Source: CAD feature listing. Evaluate the final solid. Frame: model axes, mm. A direction names the side the tool comes from. Coordinates: 2 decimals unless noted, no trailing zeros. Order: outer loops, then holes, each group sorted by start corner. A loop starts at its lowest first (then second) coordinate and runs counter-clockwise, first axis right, second up.
Item 1: Contact query for flat-ended pins moving along their axis: P1, Ø1.5, axis at x = 4.5, z = -7, coming from the -Y side; P2, Ø2, axis at x = 8, z = -6.5, coming from the +Y side; P3, Ø10, axis at x = 4.5, z = -7, coming from the -Y side. Output: stop coordinate, or through.
Item 2: Section A-A on y = -29. Return the cut outline in (x, z), then the cut area to 3 significant figures.
Item 3: Ray query, line 1 (Z direction, x = -5.5, y = -33.5); line 2 (Y direction, x = 0.25, z = 6.75); line 3 (Z direction, x = -0.25, y = -3.5). Return the intervals inside material, ascending.
Item 4: Reachability of faces 1 (the flat face through (10, 0.381, -1)), 2 (the flat face through (-10, 0.381, -1)), 3 (the flat face through (6.2, 0, 2)) from +Z, -Z, +X, -X, +Y, -Y: full face, straight path, thin tool, end or side. Return the list, or none.
Autodesk Inventor part; units mm, degrees
ref_plane "YZ Plane" through (0, 0, 0) normal (1, 0, 0) x (0, 1, 0)
ref_plane "XZ Plane" through (0, 0, 0) normal (0, 1, 0) x (-1, 0, 0)
ref_plane "XY Plane" through (0, 0, 0) normal (0, 0, 1) x (1, 0, 0)
sketch "Sketch1" plane through (0, 0, 0) normal (0, 0, 1) x (1, 0, 0)
  line L0 (0, 0) -> (6.35, 0)
  line L1 (6.35, 0) -> (6.35, -44.45)
  line L2 (6.35, -44.45) -> (0, -44.45)
  line L3 (0, -44.45) -> (0, 0)
  dimension "d0" = 12.7
  dimension "d1" = 44.45
revolve "Revolution1" add sketch "Sketch1" angle 360 about axis through (0, -44.45, 0) along (0, 1, 0)
chamfer "Chamfer1" distance 3.175 angle 45 1 edges at (-6.35, -44.45, 0)
sketch "Sketch2" plane through (0, 0, 0) normal (0, 1, 0) x (1, 0, 0)
  circle A0 centre (0, 0) radius 9.525
  point P0 (0, 0)
  dimension "d6" = 19.05
extrude "Extrusion1" add sketch "Sketch2" along normal blind 6.35
sketch "Sketch3" plane through (0, 6.35, 0) normal (0, 1, 0) x (1, 0, 0)
  line L0 (10.9985, 0) -> (5.4993, -9.525)
  line L1 (5.4993, -9.525) -> (-5.4993, -9.525)
  line L2 (-5.4993, -9.525) -> (-10.9985, 0)
  line L3 (-10.9985, 0) -> (-5.4993, 9.525)
  line L4 (-5.4993, 9.525) -> (5.4993, 9.525)
  line L5 (5.4993, 9.525) -> (10.9985, 0)
  circle A0 centre (0, 0) radius 9.525 construction
  point P0 (0, 0)
  point P1 (0, 0)
extrude "Extrusion2" add sketch "Sketch3" against normal blind 5.969
sketch "Sketch4" plane through (0, 0, 0) normal (0, 0, 1) x (1, 0, 0)
  line L0 (9.2388, 6.35) -> (10.9985, 6.35)
  line L1 (10.9985, 6.35) -> (10.9985, 5.334)
  line L2 (10.9985, 5.334) -> (9.2388, 6.35)
  line L3 (0, -1.5875) -> (0, 9.525)
  line L4 (5.4993, 0) -> (10.9985, 0) construction
  line L5 (5.4993, 6.35) -> (10.9985, 6.35) construction
  line L6 (5.4993, 6.35) -> (5.4993, 0.381) construction
  line L7 (10.9985, 6.35) -> (10.9985, 0.381) construction
  line L8 (10.9985, 6.35) -> (5.4993, 6.35)
  line L9 (8.2489, 0.381) -> (10.9985, 0.381)
  line L10 (5.4993, 0.381) -> (8.2489, 0.381)
  point P0 (0, 0)
  point P1 (16.2522, 7.9375)
  dimension "d11" = 30
  dimension "d17" = 1.016
revolve "Revolution2" cut sketch "Sketch4" angle 360 about axis through (0, -10, 0) along (0, 1, 0)
thread "Thread3"
equation "\"diameter\" = 1.8542"
equation "\"length\" = 19.05"
properties part number "Door Hinge Pin" material "Steel, Carbon"
Answer list:
1. P1: stops at y = 0
1. P2: stops at y = 6.31
1. P3: stops at y = -44.3
2. outline: circle Ø12.7 at (0, 0)
2. area: 127 mm2
3. line 1: z = -3.17 to 3.17
3. line 2: y = 0 to 6.35
3. line 3: z = -6.35 to 6.35
4. face 1: +X, -Y
4. face 2: -X, -Y
4. face 3: -Y
